Design review of the part built by this model. Coordinates are the model's own, in mm. Face numbers are marked on the shaded views. Coordinates: 2 decimals unless noted, no trailing zeros. Write each loop counter-clockwise with the first axis right and the second up, starting at its lowest first coordinate (ties: lowest second). Pieces come first, ordered by that corner, then holes. Notation, with made-up numbers: (-29.75, 11) -> (15.25, 11) arc R33 ccw to (15.25, 44) -> close; hole circle Ø8 at (-23.5, 0.5). An arc over 180 degrees is marked (long way). Answer in a Markdown table with one row per item. Add a question column.
Item 1: Take a section at A-A, the plane y = 93. Write out the cut boundary in (x, z).
Item 2: To check wall thickness, follow line 1 (X direction, y = 154, z = 0); line 2 (X direction, y = 3, z = 0); line 3 (Z direction, x = 23, y = 177.5). State the ranges of each line that lie inside material, in increasing order.
Item 3: Draft analysis for pull direction Z (two halves, no side actions). For the marked faces 1 and 2, state which applies: released by +Z, released by -Z, zero draft, split by the parting line, or undercut.
Item 4: Clearance check with flat-ended pins moving along their axes: P1, Ø10, axis at x = 24, y = 139.5, coming from the -Z side; P2, Ø3, axis at x = -18.5, y = 144.5, coming from the -Z side; P3, Ø4, axis at x = -13.5, z = -6.5, coming from the +Y side. State where each tip first meets the part, or that it passes through.
from build123d import *


with BuildPart() as part:
    # Sketch1 → Revolve1 (revolve)
    with BuildSketch(Plane.XY, mode=Mode.PRIVATE) as revolve1_sk:
        with BuildLine():
            Line((0.923731328, 2.372383803), (7.281644407, 2.372383803))
            ThreePointArc((7.281644407, 2.372383803), (7.667037893, 5.060184318), (8.614988038, 7.604627336))
            Line((8.614988038, 7.604627336), (30.062471525, 50.490436874))
            ThreePointArc((30.062471525, 50.490436874), (31.063868878, 53.252629767), (31.403731328, 56.171019692))
            Line((31.403731328, 56.171019692), (31.403731328, 230.972383803))
            Line((31.403731328, 230.972383803), (25.053731328, 230.972383803))
            Line((25.053731328, 230.972383803), (25.053731328, 57.670337636))
            ThreePointArc((25.053731328, 57.670337636), (24.713868878, 54.751947711), (23.712471525, 51.989754818))
            Line((23.712471525, 51.989754818), (2.264991132, 9.103951467))
            ThreePointArc((2.264991132, 9.103951467), (1.263593779, 6.341758574), (0.923731328, 3.423368649))
            Line((0.923731328, 3.423368649), (0.923731328, 2.372383803))
        make_face()
    revolve(revolve1_sk.sketch.rotate(Axis((-0.346268672, 2.373242664, 0), (0, 1, 0)), 90), axis=Axis((-0.346268672, 2.373242664, 0), (0, 1, 0)))


solid = part.part
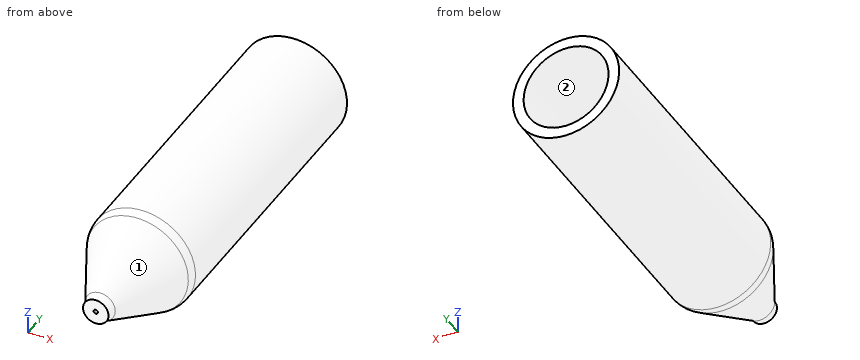
Answers:
| question | item | result |
|---|---|---|
| 1 | outline | circle Ø63.5 at (-0.35, 0); hole circle Ø50.8 at (-0.35, 0) |
| 2 | line 1 | x = -32.1 to -25.75, 25.05 to 31.4 |
| 2 | line 2 | x = -8.01 to -1.62, 0.92 to 7.32 |
| 2 | line 3 | z = -21.52 to -10.01, 10.01 to 21.52 |
| 3 | face 1 | split by the parting line |
| 3 | face 2 | undercut |
| 4 | P1 | stops at z = -25.18 |
| 4 | P2 | stops at z = -27.03 |
| 4 | P3 | stops at y = 37.22 |
